CAD build for the part. Positions are in the model's coordinates, mm. Face numbers are marked on the shaded views. A direction names the side the tool comes from. Round coordinates to 2 decimals unless told otherwise and drop trailing zeros. Loops run counter-clockwise (first coordinate to the right, second up) from the corner with the lowest first, then second, coordinate; pieces in that order, holes last.
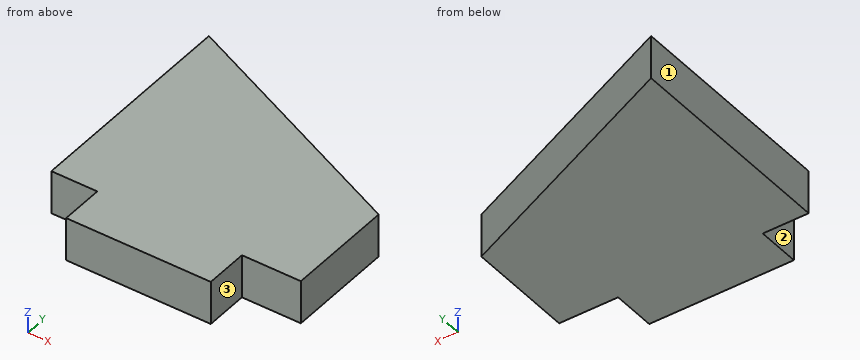
Autodesk Inventor part; units mm, degrees
ref_plane "YZ Plane" through (0, 0, 0) normal (1, 0, 0) x (0, 1, 0)
ref_plane "XZ Plane" through (0, 0, 0) normal (0, 1, 0) x (-1, 0, 0)
ref_plane "XY Plane" through (0, 0, 0) normal (0, 0, 1) x (1, 0, 0)
ref_plane "Work Plane1" through (0, 0, 0) normal (0, 0, 1) x (1, 0, 0)
sketch "Sketch1" plane through (0, 0, 0) normal (0, 0, 1) x (1, 0, 0)
  line L0 (0, 0) -> (20, 0)
  line L1 (0, 0) -> (0, -6)
  line L2 (20, -6) -> (0, -6)
  line L3 (20, 0) -> (20, -6)
  line L4 (34.15, 0) -> (34.15, 6.2)
  line L5 (34.15, 0) -> (28.15, 0)
  line L6 (28.15, 6.2) -> (28.15, 0)
  line L7 (34.15, 6.2) -> (28.15, 6.2)
  line L8 (28.15, 15) -> (28.15, 0)
  line L9 (-7.85, 48.6) -> (-7.85, 2.8)
  line L10 (-7.85, 0) -> (28.15, 0)
  line L11 (28.15, 0) -> (28.15, 15)
  line L12 (28.15, 15) -> (-7.85, 15)
  line L13 (-7.85, 15) -> (-7.85, 0)
  line L14 (28.15, 15) -> (-7.85, 31.05)
  line L15 (-7.85, 31.05) -> (-7.85, 15)
  line L16 (-6.35, 0) -> (-6.35, 30.3813)
  point P0 (-8.95, 31.05)
  dimension "d1" = 1.5
extrude "Plate2" add sketch "Sketch1" along normal blind 6 contours L10 L16 L12 L8 L6 L0 | L0 L3 L2 L1 | L16 L14 L12
equation "\"d2\" = Thickness"
equation "\"BendRadius\" = Thickness"
equation "\"BendReliefWidth\" = Thickness"
equation "\"BendReliefDepth\" = 0.5 * Thickness"
equation "\"CornerReliefSize\" = 4 * Thickness"
equation "\"MinimumRemnant\" = 2 * Thickness"
equation "\"TransitionRadius\" = BendRadius"
equation "\"JacobiRadiusSize\" = BendRadius"
equation "\"GapSize\" = Thickness"
properties part number "tussenschotje" material "Wood (Birch)"
Item 1: Cut at C-C, the plane x = -3.5. Give the cut face in (y, z).
Answers follow:
outline: (0, 0) - (29.11, 0) - (29.11, 6) - (0, 6) - close
Item 2: Flat gauge pins, fed straight in: P1, Ø1.8, axis at x = -2, z = 3, coming from the -Y side; P2, Ø3, axis at y = -2.5, z = 3.5, coming from the +X side; P3, Ø3, axis at x = 13, y = 23.5, coming from the -Z side. Where does each tip first touch, or does it go through?
Answers follow:
P1: stops at y = 0
P2: stops at x = 20
P3: passes through
Item 3: Probe line 1 (X direction, y = -3, z = 3.85); line 2 (X direction, y = 28, z = 4.8); line 3 (Y direction, x = 6.5, z = 5.7). List the from-to ranges inside material, lowest first.
Answers follow:
line 1: x = 0 to 20
line 2: x = -6.35 to -1.01
line 3: y = -6 to 24.65
Item 4: Cut at A-A, the plane z = 2. Give the cut face in (x, y), plus the area to 3 significant figures.
Answers follow:
outline: (-6.35, 0) - (0, 0) - (0, -6) - (20, -6) - (20, 0) - (28.15, 0) - (28.15, 15) - (-6.35, 30.38) - close
area: 903 mm2
Item 5: 3-axis set-ups, long thin cutter, end or side, ignore diameter. For the marked faces 1, 2 and 3: which of +Z, -Z, +X, -X, +Y, -Y reach the whole face in a straight line?
Answers follow:
face 1: +Z, -Z, -X, +Y, -Y
face 2: +Z, -Z, -X, -Y
face 3: +Z, -Z, +X, -Y
Item 6: Cut at B-B, the plane y = -2. Give the cut face in (x, z), plus the area to 3 significant figures.
Answers follow:
outline: (0, 0) - (20, 0) - (20, 6) - (0, 6) - close
area: 120 mm2
